The figure shows three views and two pictorial views of one solid part (mm, origin at its lowest corner). Answer the questions. Round coordinates to 2 decimals unless told otherwise and drop trailing zeros. Order: outer loops, then holes, each group sorted by start corner. A loop starts at its lowest first (then second) coordinate and runs counter-clockwise, first axis right, second up. Notation, with made-up numbers: (-6, 60) - (27, 60) arc R26 ccw to (27, 81) - close; hole circle Ø4 at (27, 13). An arc over 180 degrees is marked (long way). Answer in a Markdown table with one row per item.
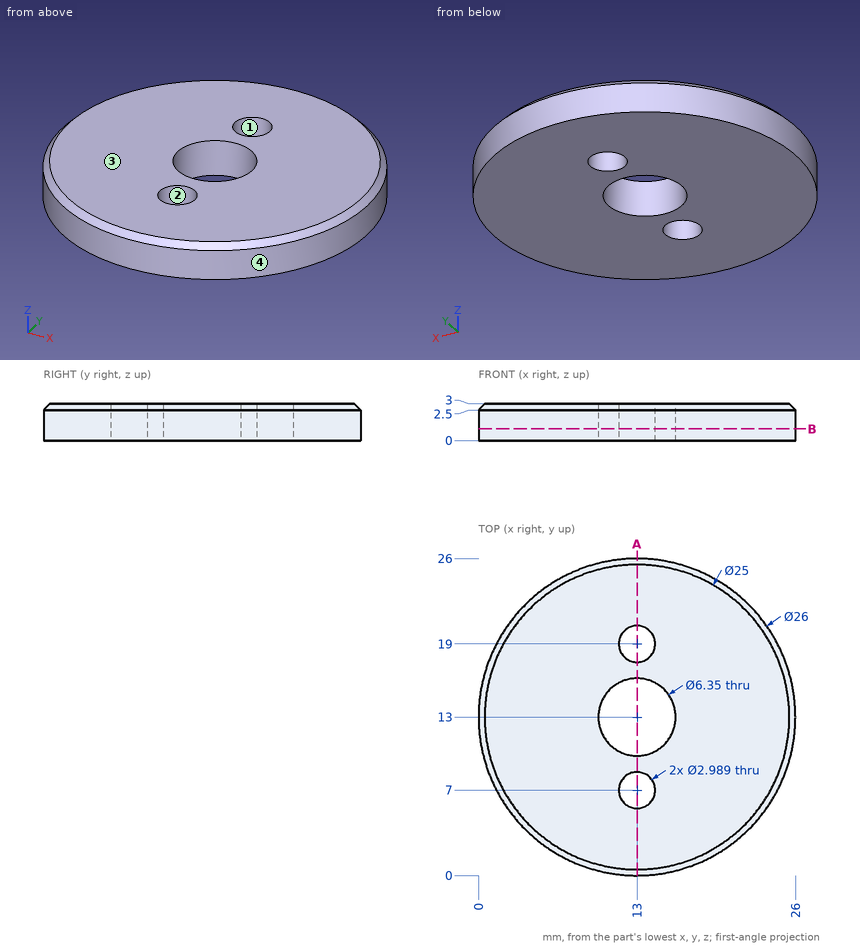
1) Find section A-A, the plane x = 13. Give the vertices of the cut face in (y, z) (1 decimal).
Filled in:
| item | result |
|---|---|
| outline | (0, 0) - (5.5, 0) - (5.5, 3) - (0.5, 3) - (0, 2.5) - close; (8.5, 0) - (9.8, 0) - (9.8, 3) - (8.5, 3) - close; (16.2, 0) - (17.5, 0) - (17.5, 3) - (16.2, 3) - close; (20.5, 0) - (26, 0) - (26, 2.5) - (25.5, 3) - (20.5, 3) - close |
2) The mould has two halves that part along X. Classify the marked faces 1, 2, 3 and 4: released by +X, released by -X, zero draft, split by the parting line, or undercut.
Filled in:
| item | result |
|---|---|
| face 1 | undercut |
| face 2 | undercut |
| face 3 | zero draft |
| face 4 | split by the parting line |
3) Find section B-B, the plane z = 0.95. Give the number of separate pieces and of enclosed holes in the cut face, then the cut area to 3 significant figures.
Filled in:
| item | result |
|---|---|
| separate pieces | 1 |
| enclosed holes | 3 |
| area | 485 mm^2 |
4) Find the intervals of material crossed by probe 1 along Y at (x, z) = (13, 0.85) (1 decimal); probe 2 along X at (y, z) = (14, 1); probe 3 along X at (y, z) = (12.75, 1.45) (1 decimal), in increasing order. Write a range as from..to.
Filled in:
| item | result |
|---|---|
| probe 1 | y = 0..5.5, 8.5..9.8, 16.2..17.5, 20.5..26 |
| probe 2 | x = 0.04..9.99, 16.01..25.96 |
| probe 3 | x = 0..9.8, 16.2..26 |
5) This flat-tipped pin is pushed along its axis until it touches: pin 1 (1.5 mm diameter, centred on y = 12, z = 1, fed in from +X). Where does it stop, or does it pass through?
Filled in:
| item | result |
|---|---|
| pin 1 | stops at x = 26 |
